```python
from build123d import *

# Parameters (mm, degrees)
F1_DEPTH = 7


with BuildPart() as f1:
    # F0 (on Top) → F1 (new body)
    with BuildSketch(Plane.XY):
        with BuildLine():
            ThreePointArc((-20.1769145362, 18), (-21.488385021, 23.2088766383), (-25.110077415, 27.1757009184))
            ThreePointArc((-25.110077415, 27.1757009184), (-29.7748571992, 28.9102811707), (-34.7266408906, 28.4115053095))
            ThreePointArc((-34.7266408906, 28.4115053095), (-42.0199383865, 19.8517110421), (-37.9807286986, 9.3566145033))
            ThreePointArc((-37.9807286986, 9.3566145033), (-36.4240480944, 8.3321362534), (-34.7167699787, 7.585134497))
            ThreePointArc((-34.7167699787, 7.585134497), (-28.3109335724, 7.379917462), (-22.878035033, 10.7799862195))
            ThreePointArc((-22.878035033, 10.7799862195), (-22.7206495749, 10.9739866522), (-22.5587647959, 11.1642487573))
            ThreePointArc((-22.5587647959, 11.1642487573), (-20.9409937058, 13.9718583996), (-20.2114514306, 17.1290126994))
            ThreePointArc((-20.2114514306, 17.1290126994), (-20.1855521511, 17.5641641149), (-20.1769145362, 18))
        make_face()
        Polygon((-27.4818728134, 24.4), (-23.7868310906, 18), (-27.4818728134, 11.6), (-34.8719562591, 11.6), (-38.5669979819, 18), (-34.8719562591, 24.4), align=None, mode=Mode.SUBTRACT)
        with BuildLine():
            ThreePointArc((-25.110077415, 27.1757009184), (-10.6130898996, 24.8635046125), (0.2578098611, 14.9977843055))
            ThreePointArc((0.2578098611, 14.9977843055), (2.8117454732, 14.7341130508), (5.2833018212, 14.0387578463))
            ThreePointArc((5.2833018212, 14.0387578463), (-0.1548013079, 22.1020653498), (-7.9047923881, 27.9780786067))
            ThreePointArc((-7.9047923881, 27.9780786067), (-9.7736896067, 28.8795995701), (-11.7009340456, 29.6485246209))
            ThreePointArc((-11.7009340456, 29.6485246209), (-23.3386442583, 31.3540820363), (-34.7266408906, 28.4115053095))
            ThreePointArc((-34.7266408906, 28.4115053095), (-29.7748571992, 28.9102811707), (-25.110077415, 27.1757009184))
        make_face()
        with BuildLine():
            ThreePointArc((-10.4801536135, -3.3743859051), (-8.1623807228, 7.3888863123), (2.3177728907, 10.7632722175))
            ThreePointArc((2.3177728907, 10.7632722175), (1.3849026925, 12.9277700022), (0.2578098611, 14.9977843055))
            ThreePointArc((0.2578098611, 14.9977843055), (-2.2008314196, 14.8376662943), (-4.6000937333, 14.2772244377))
            ThreePointArc((-4.6000937333, 14.2772244377), (-6.3822716771, 13.5744837191), (-8.0603476006, 12.6503279229))
            ThreePointArc((-8.0603476006, 12.6503279229), (-13.6968225738, 6.1153128606), (-14.799571843, -2.4439053302))
            ThreePointArc((-14.799571843, -2.4439053302), (-14.1659889408, -4.9320135166), (-13.1173671396, -7.2756222638))
            ThreePointArc((-13.1173671396, -7.2756222638), (-11.8882285824, -5.2645240876), (-10.4801536135, -3.3743859051))
        make_face()
        with BuildLine():
            ThreePointArc((2.3177728907, 10.7632722175), (8.565593369, 6.9174207792), (11.01, 0))
            ThreePointArc((11.01, 0), (10.273458808, -3.9593110665), (8.1623807228, -7.3888863123))
            ThreePointArc((8.1623807228, -7.3888863123), (10.5033258899, -7.6632459146), (12.8595572786, -7.7221620418))
            ThreePointArc((12.8595572786, -7.7221620418), (13.9502116536, -5.5128572283), (14.6644859253, -3.154814186))
            ThreePointArc((14.6644859253, -3.154814186), (14.9158856405, -1.5863024808), (15, 0))
            ThreePointArc((15, 0), (14.9964193596, 0.327729144), (14.9856791478, 0.655301824))
            ThreePointArc((14.9856791478, 0.655301824), (12.1444275762, 8.8041398697), (5.2833018212, 14.0387578463))
            ThreePointArc((5.2833018212, 14.0387578463), (2.8117454732, 14.7341130508), (0.2578098611, 14.9977843055))
            ThreePointArc((0.2578098611, 14.9977843055), (1.3849026925, 12.9277700022), (2.3177728907, 10.7632722175))
        make_face()
        with BuildLine():
            ThreePointArc((12.8595572786, -7.7221620418), (10.5033258899, -7.6632459146), (8.1623807228, -7.3888863123))
            ThreePointArc((8.1623807228, -7.3888863123), (-2.3177728907, -10.7632722175), (-10.4801536135, -3.3743859051))
            ThreePointArc((-10.4801536135, -3.3743859051), (-11.8882285824, -5.2645240876), (-13.1173671396, -7.2756222638))
            ThreePointArc((-13.1173671396, -7.2756222638), (-11.749380234, -9.324809066), (-10.0643921919, -11.1224102517))
            ThreePointArc((-10.0643921919, -11.1224102517), (-8.5647119055, -12.3144512657), (-6.9253315472, -13.3056297469))
            ThreePointArc((-6.9253315472, -13.3056297469), (1.5523949975, -14.9194527303), (9.5162700219, -11.5948525161))
            ThreePointArc((9.5162700219, -11.5948525161), (11.3542434676, -9.8020995342), (12.8595572786, -7.7221620418))
        make_face()
        with BuildLine():
            ThreePointArc((-10.9798086535, -35.3338153916), (-16.2258816717, -21.6229577719), (-13.1173671396, -7.2756222638))
            ThreePointArc((-13.1173671396, -7.2756222638), (-14.1659889408, -4.9320135166), (-14.799571843, -2.4439053302))
            ThreePointArc((-14.799571843, -2.4439053302), (-19.0635494151, -11.1850945401), (-20.2773306285, -20.8347903231))
            ThreePointArc((-20.2773306285, -20.8347903231), (-20.1236220755, -22.9040632731), (-19.8259084836, -24.957568442))
            ThreePointArc((-19.8259084836, -24.957568442), (-15.4841094266, -35.8888998357), (-7.2417649124, -44.2799058541))
            ThreePointArc((-7.2417649124, -44.2799058541), (-10.1496093248, -40.2409233139), (-10.9798086535, -35.3338153916))
        make_face()
        with BuildLine():
            ThreePointArc((-8.0603476006, 12.6503279229), (-6.3822716771, 13.5744837191), (-4.6000937333, 14.2772244377))
            ThreePointArc((-4.6000937333, 14.2772244377), (-11.9690338946, 18.0939285598), (-20.2114514306, 17.1290126994))
            ThreePointArc((-20.2114514306, 17.1290126994), (-20.9409937058, 13.9718583996), (-22.5587647959, 11.1642487573))
            ThreePointArc((-22.5587647959, 11.1642487573), (-15.6028763872, 14.7689652749), (-8.0603476006, 12.6503279229))
        make_face()
        with BuildLine():
            ThreePointArc((36.0898860685, 8.1581144732), (26.8389715713, -3.2405468406), (12.8595572786, -7.7221620418))
            ThreePointArc((12.8595572786, -7.7221620418), (11.3542434676, -9.8020995342), (9.5162700219, -11.5948525161))
            ThreePointArc((9.5162700219, -11.5948525161), (19.218350723, -10.9169708097), (28.1821230165, -7.1432882836))
            ThreePointArc((28.1821230165, -7.1432882836), (29.8973116822, -5.9755362969), (31.5268425292, -4.6909561789))
            ThreePointArc((31.5268425292, -4.6909561789), (38.8227536849, 4.5348177995), (41.9684058031, 15.8684005447))
            ThreePointArc((41.9684058031, 15.8684005447), (39.924466524, 11.3306421432), (36.0898860685, 8.1581144732))
        make_face()
        with BuildLine():
            ThreePointArc((24.9398858547, 8.9391240365), (30.4082951127, 7.0268863042), (36.0898860685, 8.1581144732))
            ThreePointArc((36.0898860685, 8.1581144732), (39.924466524, 11.3306421432), (41.9684058031, 15.8684005447))
            ThreePointArc((41.9684058031, 15.8684005447), (42.1246632531, 16.9291134362), (42.1769145362, 18))
            ThreePointArc((42.1769145362, 18), (37.3446399002, 27.1081921277), (27.0934302026, 28.2139686556))
            ThreePointArc((27.0934302026, 28.2139686556), (25.4278657104, 27.3780828317), (23.9273041549, 26.2730374904))
            ThreePointArc((23.9273041549, 26.2730374904), (20.5466627861, 20.8280289476), (20.774759435, 14.4229664175))
            ThreePointArc((20.774759435, 14.4229664175), (20.8640760091, 14.1896663962), (20.9479054359, 13.9543390126))
            ThreePointArc((20.9479054359, 13.9543390126), (22.570481165, 11.1495033299), (24.9398858547, 8.9391240365))
        make_face()
        Polygon((34.8719562591, 24.4), (38.5669979819, 18), (34.8719562591, 11.6), (27.4818728134, 11.6), (23.7868310906, 18), (27.4818728134, 24.4), align=None, mode=Mode.SUBTRACT)
        with BuildLine():
            ThreePointArc((-4.7284344241, -26.0681367359), (-9.1186855075, -29.8477992055), (-10.9798086535, -35.3338153916))
            ThreePointArc((-10.9798086535, -35.3338153916), (-10.1496093248, -40.2409233139), (-7.2417649124, -44.2799058541))
            ThreePointArc((-7.2417649124, -44.2799058541), (3.8178831222, -46.3161896292), (10.887298496, -37.5705831589))
            ThreePointArc((10.887298496, -37.5705831589), (10.9717884471, -36.7873107849), (11, -36))
            ThreePointArc((11, -36), (10.9472399275, -34.9239247384), (10.7894658239, -33.8581719874))
            ThreePointArc((10.7894658239, -33.8581719874), (7.7642707863, -28.2079464095), (2.1032755979, -25.202952637))
            ThreePointArc((2.1032755979, -25.202952637), (1.8565735658, -25.1636530484), (1.61085936, -25.1185877699))
            ThreePointArc((1.61085936, -25.1185877699), (-1.6294874593, -25.1213617295), (-4.7284344241, -26.0681367359))
        make_face()
        Polygon((3.6950417228, -42.4), (-3.6950417228, -42.4), (-7.3900834456, -36), (-3.6950417228, -29.6), (3.6950417228, -29.6), (7.3900834456, -36), align=None, mode=Mode.SUBTRACT)
        with BuildLine():
            ThreePointArc((15, 0), (14.9158856405, -1.5863024808), (14.6644859253, -3.154814186))
            ThreePointArc((14.6644859253, -3.154814186), (21.6543187343, 1.3185231315), (24.9398858547, 8.9391240365))
            ThreePointArc((24.9398858547, 8.9391240365), (22.570481165, 11.1495033299), (20.9479054359, 13.9543390126))
            ThreePointArc((20.9479054359, 13.9543390126), (20.5917373093, 6.128004686), (14.9856791478, 0.655301824))
            ThreePointArc((14.9856791478, 0.655301824), (14.9964193596, 0.327729144), (15, 0))
        make_face()
        with BuildLine():
            ThreePointArc((-6.9253315472, -13.3056297469), (-8.5647119055, -12.3144512657), (-10.0643921919, -11.1224102517))
            ThreePointArc((-10.0643921919, -11.1224102517), (-9.6852848398, -19.4124516913), (-4.7284344241, -26.0681367359))
            ThreePointArc((-4.7284344241, -26.0681367359), (-1.6294874593, -25.1213617295), (1.61085936, -25.1185877699))
            ThreePointArc((1.61085936, -25.1185877699), (-4.9888609221, -20.8969699609), (-6.9253315472, -13.3056297469))
        make_face()
        with BuildLine():
            ThreePointArc((-19.8259084836, -24.957568442), (-20.1236220755, -22.9040632731), (-20.2773306285, -20.8347903231))
            ThreePointArc((-20.2773306285, -20.8347903231), (-31.931222333, -8.87771769), (-34.7167699787, 7.585134497))
            ThreePointArc((-34.7167699787, 7.585134497), (-36.4240480944, 8.3321362534), (-37.9807286986, 9.3566145033))
            ThreePointArc((-37.9807286986, 9.3566145033), (-34.8113873846, -10.9262960202), (-19.8259084836, -24.957568442))
        make_face()
        with BuildLine():
            ThreePointArc((-11.7009340456, 29.6485246209), (-9.7736896067, 28.8795995701), (-7.9047923881, 27.9780786067))
            ThreePointArc((-7.9047923881, 27.9780786067), (8.2772821194, 32.0921085593), (23.9273041549, 26.2730374904))
            ThreePointArc((23.9273041549, 26.2730374904), (25.4278657104, 27.3780828317), (27.0934302026, 28.2139686556))
            ThreePointArc((27.0934302026, 28.2139686556), (7.9432437696, 35.6106938262), (-11.7009340456, 29.6485246209))
        make_face()
        with BuildLine():
            ThreePointArc((31.5268425292, -4.6909561789), (29.8973116822, -5.9755362969), (28.1821230165, -7.1432882836))
            ThreePointArc((28.1821230165, -7.1432882836), (23.6539402137, -23.2143908693), (10.7894658239, -33.8581719874))
            ThreePointArc((10.7894658239, -33.8581719874), (10.9472399275, -34.9239247384), (11, -36))
            ThreePointArc((11, -36), (10.9717884471, -36.7873107849), (10.887298496, -37.5705831589))
            ThreePointArc((10.887298496, -37.5705831589), (26.8681436151, -24.684397806), (31.5268425292, -4.6909561789))
        make_face()
    extrude(amount=F1_DEPTH)


solid = f1.part
```
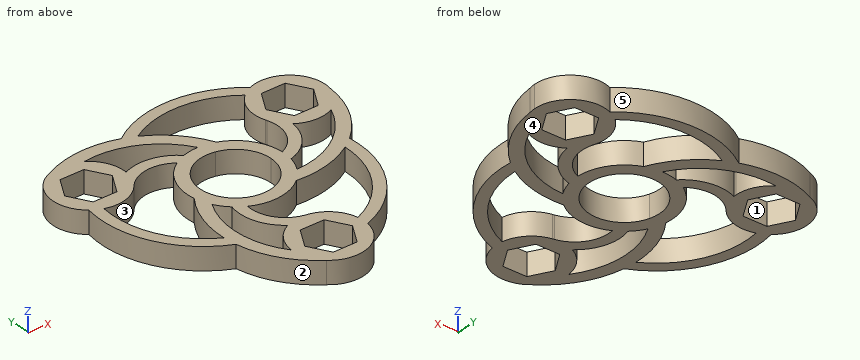
Design review of the part built by this model. Coordinates are the model's own, in mm. Face numbers are marked on the shaded views. A direction names the side the tool comes from. Give positions to 0.01 mm unless a question says otherwise; leave off trailing zeros. Order: outer loops, then holes, each group sorted by start corner. A loop starts at its lowest first (then second) coordinate and runs counter-clockwise, first axis right, second up. Notation, with made-up numbers: (-35.5, 65.25) - (-12.5, 65.25) arc R15 cw to (-12.5, 86.25) - close; hole circle Ø4 at (39, -19.75). An arc over 180 degrees is marked (long way). Use a Markdown table: item, result. Add a question column.
(1) Wall thickness on probe 1 along Y at (x, z) = (1.5, 2.5); probe 2 along Y at (x, z) = (10, 5.25); probe 3 along X at (y, z) = (13.5, 6.5): over which ranges is each line inside the solid? List them lowest first. Write a range as [from, to].
(2) Add section C-C on y = -22. Give the boundary of the cut face in (x, z).
(3) Add section A-A on y = 3.5. Give the boundary of the cut face in (x, z).
(4) Add section D-D on z = 2. Give the number of separate pieces and of enclosed holes in the cut face, then the cut area to 3 significant figures.
(5) Clearance check with flat-ended pins moving along their axes: P1, Ø2, axis at y = -22, z = 2.5, coming from the -X side; P2, Ø1.5, axis at x = -31, z = 3, coming from the -Y side; P3, Ø2, axis at y = -20, z = 3.5, coming from the -X side. State where each tip first meets the part, or that it passes through.
(6) Add section B-B on x = -30. Give the boundary of the cut face in (y, z), then the cut area to 3 significant figures.
(7) Machinability: for the marked faces 1 and 2, which of the approach directions +Z, -Z, +X, -X, +Y, -Y give a long, thin tool a straight path to every point of the face, cutting with its end or side? Answer none if there is none.
(8) Mouldability with a two-part tool opening along Y and no side actions: class the marked faces 3, 4 and 5 as +Y half, -Y half, draft (parallel to the pull), parting line (faces both ways), or undercut.
Report:
| question | item | result |
|---|---|---|
| 1 | probe 1 | y = [-46.9, -42.4], [-29.6, -25.1], [-14.92, -10.91], [10.91, 20.2], [31.63, 35.19] |
| 1 | probe 2 | y = [-40.58, -31.42], [-11.64, -4.61], [4.61, 11.18], [31.95, 35.47] |
| 1 | probe 3 | x = [-41.21, -35.97], [-26.38, -19.66], [-9.37, 6.54], [21.09, 26.38], [35.97, 41.7] |
| 2 | outline | (-25.04, 0) - (-16.19, 0) - (-16.19, 7) - (-25.04, 7) - close; (-8.45, 0) - (-4.07, 0) - (-4.07, 7) - (-8.45, 7) - close; (24.4, 0) - (28.38, 0) - (28.38, 7) - (24.4, 7) - close |
| 3 | outline | (-38.47, 0) - (-34.97, 0) - (-34.97, 7) - (-38.47, 7) - close; (-14.59, 0) - (-10.44, 0) - (-10.44, 7) - (-14.59, 7) - close; (10.44, 0) - (14.59, 0) - (14.59, 7) - (10.44, 7) - close; (18.91, 0) - (23.18, 0) - (23.18, 7) - (18.91, 7) - close; (33.57, 0) - (38.27, 0) - (38.27, 7) - (33.57, 7) - close |
| 4 | separate pieces | 1 |
| 4 | enclosed holes | 10 |
| 4 | area | 2,040 mm² |
| 5 | P1 | stops at x = -26.39 |
| 5 | P2 | stops at y = -17.41 |
| 5 | P3 | stops at x = -28.7 |
| 6 | outline | (-17.69, 0) - (-12.12, 0) - (-12.12, 7) - (-17.69, 7) - close; (7.06, 0) - (11.6, 0) - (11.6, 7) - (7.06, 7) - close; (24.4, 0) - (30.23, 0) - (30.23, 7) - (24.4, 7) - close |
| 6 | area | 112 mm² |
| 7 | face 1 | +Z, -Z |
| 7 | face 2 | +Z, -Z, -X, -Y |
| 8 | face 3 | undercut |
| 8 | face 4 | draft |
| 8 | face 5 | +Y half |
